Could you check a few things on this model? Use its own coordinates, in mm. A direction names the side the tool comes from. Give positions to 0.01 mm unless a question says otherwise; leave off trailing zeros. Loops run counter-clockwise (first coordinate to the right, second up) from the corner with the lowest first, then second, coordinate; pieces in that order, holes last.
1. For P1, Ø3, axis at x = 2, y = -7, coming from the -Z side; P2, Ø4, axis at x = -1, y = -1.5, coming from the -Z side; P3, Ø1.5, axis at x = -2, y = -3, coming from the +Z side; P4, Ø4, axis at x = -3, y = -5.5, coming from the -Z side, each with a flat end and sliding along its axis, tell me the tip position at first contact or that it passes through.
2. Imagine slicing it at C-C (y = 0.75). List the corners of the cut face in (x, z) for me, plus the area to 3 significant figures.
3. Imagine slicing it at D-D (y = -1.25). List the corners of the cut face in (x, z) for me.
4. Imagine slicing it at B-B (x = 0). List the corners of the cut face in (y, z) for me, plus the area to 3 significant figures.
5. I need wall thicknesses on line 1 along X through (y, z) = (1.65, 0); line 2 along Y through (x, z) = (0.75, 3.5); line 3 along X through (y, z) = (1, -1.75). Which ranges of each line are inside material? Lowest first, please.
6. Imagine slicing it at A-A (z = 0). List the corners of the cut face in (x, y) for me.
7. Thinking about a two-plate mould opening in X: for faces 1 (the flat face through (0, 0, 0)), 2 (the flat face through (-3, 2.2, 2)), 3 (the cylindrical face through (-2.44, -4.94, 0.54)), which applies, +X half, -X half, draft (parallel to the pull), parting line (faces both ways), or undercut?
8. For faces 4 (the cylindrical face through (0.931, 1.085, 2.957)), 5 (the flat face through (2, -1, -2)), 6 (the flat face through (0, -9, 0)), which set-ups out of +Z, -Z, +X, -X, +Y, -Y let a thin tool reach every point of the face, with its end or its side?
```python
from build123d import *

# Parameters (mm, degrees)
ESQUISSE1_R        = 4
ESQUISSE1_R_2      = 3.1
BOSS_EXTRU_1_DEPTH = 2.2
BOSS_EXTRU_2_START = 1
ESQUISSE2_R        = 4
BOSS_EXTRU_2_DEPTH = 1
ESQUISSE3_R        = 2.5
BOSS_EXTRU_3_DEPTH = 8


with BuildPart() as part:
    # Esquisse1 → Boss.-Extru.1 (new body)
    with BuildSketch(Plane(origin=(0, 0, 0), x_dir=(1, 0, 0), z_dir=(0, 1, 0))):
        with Locations(Location((0, 0, 0), (0, 0, 270))):
            Circle(ESQUISSE1_R)
        with Locations(Location((0, 0, 0), (0, 0, 270))):
            Circle(ESQUISSE1_R_2, mode=Mode.SUBTRACT)
    extrude(amount=BOSS_EXTRU_1_DEPTH)

    # Esquisse2 → Boss.-Extru.2 (add)
    with BuildSketch(Plane.XZ.offset(BOSS_EXTRU_2_START)):
        with Locations(Location((0, 0, 0), (0, 0, 270))):
            Circle(ESQUISSE2_R)
    extrude(amount=-BOSS_EXTRU_2_DEPTH)

    # Esquisse3 → Boss.-Extru.3 (add)
    with BuildSketch(Plane.XZ.offset(1)):
        with Locations(Location((0, 0, 0), (0, 0, 270))):
            Circle(ESQUISSE3_R)
    extrude(amount=BOSS_EXTRU_3_DEPTH)


solid = part.part
```
Derived:
1. P1: stops at z = -2.45
1. P2: stops at z = -4
1. P3: stops at z = 2.17
1. P4: stops at z = -2.29
2. outline: circle Ø8 at (0, 0); hole circle Ø6.2 at (0, 0)
2. area: 20.1 mm2
3. outline: circle Ø5 at (0, 0)
4. outline: (-9, -2.5) - (-1, -2.5) - (-1, -4) - (2.2, -4) - (2.2, -3.1) - (0, -3.1) - (0, 3.1) - (2.2, 3.1) - (2.2, 4) - (-1, 4) - (-1, 2.5) - (-9, 2.5) - close
4. area: 52.0 mm2
5. line 1: x = -4 to -3.1, 3.1 to 4
5. line 2: y = -1 to 2.2
5. line 3: x = -3.6 to -2.56, 2.56 to 3.6
6. outline: (-4, -1) - (-2.5, -1) - (-2.5, -9) - (2.5, -9) - (2.5, -1) - (4, -1) - (4, 2.2) - (3.1, 2.2) - (3.1, 0) - (-3.1, 0) - (-3.1, 2.2) - (-4, 2.2) - close
7. face 1: undercut
7. face 2: draft
7. face 3: parting line
8. face 4: +Y
8. face 5: -Y
8. face 6: +Z, -Z, +X, -X, -Y
